Study the drawing (mm; zero at the part's minimum x, y, z) and answer. A direction names the side the tool comes from. Give positions to 0.01 mm unless a question says otherwise; leave off trailing zeros. Order: outer loops, then holes, each group sorted by start corner. A loop starts at its lowest first (then second) coordinate and runs counter-clockwise, first axis right, second up. Notation, with made-up numbers: (44.25, 3) - (54.25, 3) arc R21 ccw to (54.25, 9) - close; hole circle Ø3 at (-16, -27). An arc over 180 degrees is marked (long way). Write each question's results on one line, items separated by ' | '. Start each with the question number.
Q1. Flat-ended cylindrical pins translate along their axes: P1, Ø6, axis at y = 16, z = 3, coming from the -X side; P2, Ø3, axis at y = 12, z = 5.5, coming from the +X side. Find the tip coordinate at first contact, or state that the pin passes through.
Q2. Find section C-C on x = 6. Give the vertices of the cut face in (y, z), and give its area (3 significant figures).
Q3. A tool of negligible diameter and unlimited length cuts with its end or side. For the marked faces 1, 2 and 3, from which of +Z, -Z, +X, -X, +Y, -Y can it reach the whole face along a straight path? Write none if from no direction.
Q4. For a pull along Z with two mould halves and no side action, classify the marked faces 4, 5 and 6 as +Z half, -Z half, draft (parallel to the pull), parting line (faces both ways), or undercut.
Q5. Find the intervals of material crossed by line 1 along Y through (x, z) = (2, 4.25); line 2 along Z through (x, y) = (6.25, 39.5); line 3 along Y through (x, z) = (7, 5), in increasing order. Write a range as from..to.
Q6. Find section D-D on y = 40.5. Give the vertices of the cut face in (x, z), and give its area (3 significant figures).
Q7. Find section B-B on z = 6. Give the vertices of the cut face in (x, y), and give its area (3 significant figures).
Q8. Find section A-A on y = 48.5. Give the vertices of the cut face in (x, z).
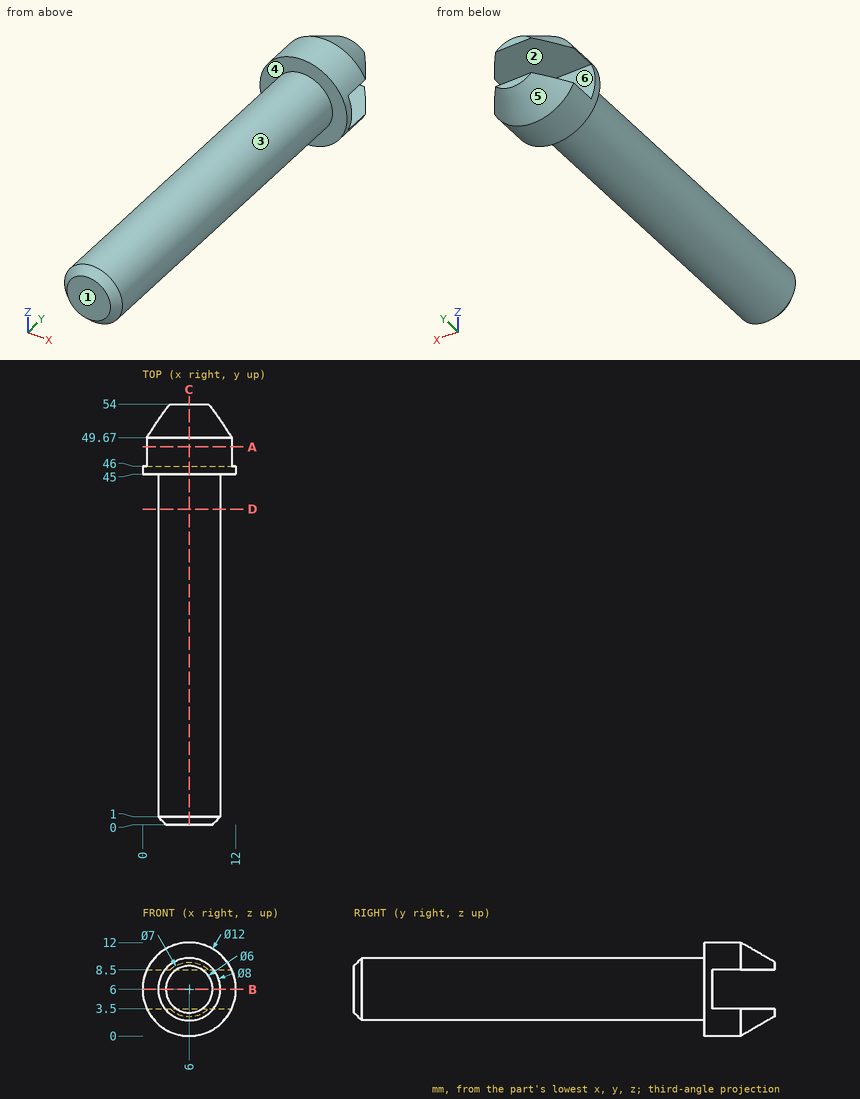
Working result:
1) P1: x = 2 | P2: x = 10
2) outline: (0, 3) - (1, 2) - (45, 2) - (45, 0) - (49.67, 0) - (54, 2.5) - (54, 3.5) - (46, 3.5) - (46, 8.5) - (54, 8.5) - (54, 9.5) - (49.67, 12) - (45, 12) - (45, 10) - (1, 10) - (0, 9) - close | area: 416 mm²
3) face 1: +Z, -Z, +X, -X, -Y | face 2: +X, -X, +Y | face 3: -Y
4) face 4: draft | face 5: -Z half | face 6: undercut
5) line 1: 45..46 | line 2: 2.01..9.99 | line 3: 0..46
6) outline: circle Ø8 at (6, 6) | area: 50.3 mm²
7) outline: (0, 45) - (2, 45) - (2, 1) - (3, 0) - (9, 0) - (10, 1) - (10, 45) - (12, 45) - (12, 46) - (0, 46) - close | area: 371 mm²
8) outline: (0.55, 3.5) arc R6 ccw to (11.45, 3.5) - close; (0.55, 8.5) - (11.45, 8.5) arc R6 ccw to start
